Autodesk Inventor part; units mm, degrees
ref_plane "BODY_N_XY" through (61, 0, 0) normal (0, 0, -1) x (1, 0, 0)
ref_plane "BODY_N_YZ" through (61, 0, 0) normal (1, 0, 0) x (0, -1, 0)
ref_plane "BODY_N_ZX" through (61, 0, 0) normal (0, -1, 0) x (0, 0, -1)
sketch "Sketch_8" plane through (0, 0, 0) normal (0, 0, 1) x (1, 0, 0)
  line L0 (0, 0) -> (-8, 0)
  line L1 (-8, 0) -> (-8, 3.3865)
  line L2 (-8, 3.3865) -> (-7.3865, 4)
  line L3 (-7.3865, 4) -> (0, 4)
  line L4 (0, 4) -> (0, 0)
  line L5 (0, 0) -> (-8, 0)
revolve "Revolution1" add sketch "Sketch_8" angle 360 about axis through (0, 0, 0) along (1, 0, 0)
thread "Thread1"
sketch "Sketch_9" plane through (0, 0, 0) normal (1, 0, 0) x (0, 0, -1)
  line L0 (-6, 3.6056) -> (-6, -3.6056)
  arc A0 (-6, -3.6056) -> (-3.6056, -6) centre (0, 0) ccw
  line L1 (-3.6056, -6) -> (3.6056, -6)
  arc A1 (3.6056, -6) -> (6, -3.6056) centre (0, 0) ccw
  line L2 (6, -3.6056) -> (6, 3.6056)
  arc A2 (6, 3.6056) -> (3.6056, 6) centre (0, 0) ccw
  line L3 (3.6056, 6) -> (-3.6056, 6)
  arc A3 (-3.6056, 6) -> (-6, 3.6056) centre (0, 0) ccw
extrude "Extrusion1" add sketch "Sketch_9" along normal blind 12.5
sketch "Sketch_6" plane through (12.5, 0, 0) normal (1, 0, 0) x (0, 0, -1)
  circle A0 centre (0, 0) radius 5.5
extrude "Extrusion2" add sketch "Sketch_6" along normal blind 39
sketch "Sketch_10" plane through (51.5, 0, 0) normal (1, 0, 0) x (0, 0, -1)
  line L0 (-6, 3.6056) -> (-6, -3.6056)
  arc A0 (-6, -3.6056) -> (-3.6056, -6) centre (0, 0) ccw
  line L1 (-3.6056, -6) -> (3.6056, -6)
  arc A1 (3.6056, -6) -> (6, -3.6056) centre (0, 0) ccw
  line L2 (6, -3.6056) -> (6, 3.6056)
  arc A2 (6, 3.6056) -> (3.6056, 6) centre (0, 0) ccw
  line L3 (3.6056, 6) -> (-3.6056, 6)
  arc A3 (-3.6056, 6) -> (-6, 3.6056) centre (0, 0) ccw
extrude "Extrusion3" add sketch "Sketch_10" along normal blind 9.5
sketch "Sketch7_ALT_Drilling_1" plane through (0, 0, 0) normal (0, 0, 1) x (1, 0, 0)
  line L0 (8, 6) -> (8, 1)
  line L1 (8, -0.1934) -> (5.933, 1)
  line L2 (5.933, 1) -> (5.933, 5.567)
  line L3 (5.933, 5.567) -> (5.5, 6)
  line L4 (5.5, 6) -> (8, 6)
  line L5 (8, 6) -> (8, -0.1934)
revolve "Revolution2" cut sketch "Sketch7_ALT_Drilling_1" angle 360 about axis through (8, 6, 0) along (0, 1, 0)
thread "Thread2"
sketch "Sketch_7_ALT_Drilling_2" plane through (0, 0, 0) normal (0, 0, 1) x (1, 0, 0)
  line L0 (56, 6) -> (56, 1)
  line L1 (56, -0.1934) -> (53.933, 1)
  line L2 (53.933, 1) -> (53.933, 5.567)
  line L3 (53.933, 5.567) -> (53.5, 6)
  line L4 (53.5, 6) -> (56, 6)
  line L5 (56, 6) -> (56, -0.1934)
revolve "Revolution3" cut sketch "Sketch_7_ALT_Drilling_2" angle 360 about axis through (56, 6, 0) along (0, 1, 0)
thread "Thread3"
sketch "Sketch_16_ALT_Drilling_3" plane through (0, 0, 0) normal (0, 0, 1) x (1, 0, 0)
  line L0 (32.5, 0) -> (-8, 0)
  line L1 (-8, 0) -> (-8, 2)
  line L2 (-8, 2) -> (12.5, 2)
  line L3 (12.5, 2) -> (12.5, 5)
  line L4 (12.5, 5) -> (32.5, 5)
  line L5 (32.5, 5) -> (32.5, 0)
  line L6 (32.5, 0) -> (-8, 0)
revolve "Revolution4" cut sketch "Sketch_16_ALT_Drilling_3" angle 360 about axis through (32.5, 0, 0) along (1, 0, 0)
ref_plane "BODY_N_XY" through (61, 0, 0) normal (0, 0, -1) x (1, 0, 0)
ref_plane "BODY_N_YZ" through (61, 0, 0) normal (1, 0, 0) x (0, -1, 0)
ref_plane "BODY_N_ZX" through (61, 0, 0) normal (0, -1, 0) x (0, 0, -1)
ref_plane "NUT2_XY" through (61, 0, 0) normal (1, 0, 0) x (0, 0, -1)
ref_plane "NUT2_YZ" through (61, 0, 0) normal (0, 0, -1) x (0, 1, 0)
ref_plane "NUT2_ZX" through (61, 0, 0) normal (0, 1, 0) x (1, 0, 0)
ref_plane "SW1_XY" through (17, 0, 0) normal (1, 0, 0) x (0, 0, -1)
ref_plane "SW1_YZ" through (17, 0, 0) normal (0, 0, -1) x (0, 1, 0)
ref_plane "SW1_ZX" through (17, 0, 0) normal (0, 1, 0) x (1, 0, 0)
ref_plane "SW2_XY" through (47, 0, 0) normal (-1, 0, 0) x (0, 0, -1)
ref_plane "SW2_YZ" through (47, 0, 0) normal (0, 0, -1) x (0, -1, 0)
ref_plane "SW2_ZX" through (47, 0, 0) normal (0, -1, 0) x (-1, 0, 0)
ref_plane "SW_R1_XY" through (17, -11, 0) normal (1, 0, 0) x (0, 0, -1)
ref_plane "SW_R1_YZ" through (17, -11, 0) normal (0, 0, -1) x (0, 1, 0)
ref_plane "SW_R1_ZX" through (17, -11, 0) normal (0, 1, 0) x (1, 0, 0)
ref_plane "SW_R2_XY" through (47, -11, 0) normal (-1, 0, 0) x (0, 0, -1)
ref_plane "SW_R2_YZ" through (47, -11, 0) normal (0, 0, -1) x (0, -1, 0)
ref_plane "SW_R2_ZX" through (47, -11, 0) normal (0, -1, 0) x (-1, 0, 0)
ref_plane "body_XY" through (0, 0, 0) normal (1, 0, 0) x (0, 0, -1)
ref_plane "body_YZ" through (0, 0, 0) normal (0, 0, -1) x (0, 1, 0)
ref_plane "body_ZX" through (0, 0, 0) normal (0, 1, 0) x (1, 0, 0)
properties part number "CJ2B10-15Z(0_0)_BODY"
Can you work these out from the model? Positions are in its coordinate system, mm. A direction names the side the tool comes from. Round coordinates to 2 decimals unless told otherwise and drop trailing zeros. Order: outer loops, then holes, each group sorted by start corner. A loop starts at its lowest first (then second) coordinate and runs counter-clockwise, first axis right, second up. Notation, with made-up numbers: (-24, 19) -> (21, 19) arc R24 ccw to (21, 57) -> close; hole circle Ø4 at (16, -38). An arc over 180 degrees is marked (long way). Return JSON: item names as keys, results as strings. Group by question number.
1. If we section it at C-C, the plane x = 18.5: Write out the boundary of the cut face in (y, z), then the cut area to 3 significant figures.
2. Which directions (+Z, -Z, +X, -X, +Y, -Y) give clear straight access to the entire face, cutting with the end or side of a thin tool? Please do faces 4 (the face through (22.64, -1.08, -4.88)), 5 (the face through (2, -2, 0)), 6 (the face through (10.065, 3.315, 0.091)).
3. If we section it at A-A, the plane x = 1: Write out the boundary of the cut face in (y, z).
4. We'd pull the mould along Z, two halves only. Please class faces 1 (the face through (51.5, -5, 3)), 2 (the face through (58.065, 3.315, 0.091)), 3 (the face through (6.2, -5, 4.9)): released by +Z, released by -Z, zero draft, split by the parting line, or undercut.
5. If we section it at B-B, the plane x = 36: Write out the boundary of the cut face in (y, z).
6. I need wall thicknesses on line 1 (X direction, y = -2.75, z = -0.25); line 2 (X direction, y = -0.5, z = -4); line 3 (Y direction, x = 28, z = -0.25). Which ranges of each line are inside material? Lowest first, please. Write a range as [from, to].
7. Will these pins go through, and if not, where does the flat tip stop? pin 1 (5 mm diameter, centred on x = 37.5, z = -4.5, fed in from -Y); pin 2 (5 mm diameter, centred on x = 20, y = -1.5, fed in from +Z); pin 3 (1.5 mm diameter, centred on x = 48.5, z = 1, fed in from +Y).
Output values:
{
 "1": {"outline": "circle Ø11 at (0, 0); hole circle Ø10 at (0, 0)", "area": "16.5 mm²"},
 "2": {"face 4": "none", "face 5": "-X", "face 6": "+Y"},
 "3": {"outline": "(-6, -3.61) arc R7 ccw to (-3.61, -6) -> (3.61, -6) arc R7 ccw to (6, -3.61) -> (6, 3.61) arc R7 ccw to (3.61, 6) -> (-3.61, 6) arc R7 ccw to (-6, 3.61) -> close; hole circle Ø4 at (0, 0)"},
 "4": {"face 1": "zero draft", "face 2": "undercut", "face 3": "released by +Z"},
 "5": {"outline": "circle Ø11 at (0, 0)"},
 "6": {"line 1": "[-8, 12.5], [32.5, 61]", "line 2": "[0, 12.5], [32.5, 61]", "line 3": "[-5.49, -4.99], [4.99, 5.49]"},
 "7": {"pin 1": "y = -5.12", "pin 2": "z = 5.5", "pin 3": "y = 5.49"}
}
